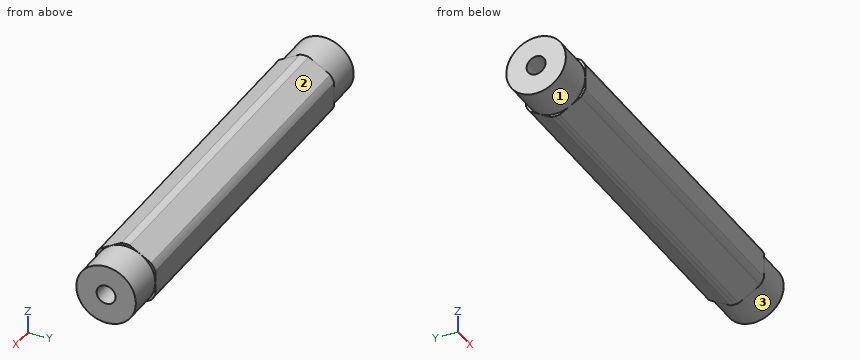
```python
from build123d import *

# Parameters (mm, degrees)
SKETCH1_R               = 2.0193
BOSS_EXTRUDE1_DEPTH     = 44.45
SKETCH2_R               = 8.89
SKETCH2_R_2             = 6.35
CUT_EXTRUDE_THIN1_DEPTH = 7.9375


with BuildPart() as part:
    # Sketch1 → Boss-Extrude1 (new, symmetric)
    with BuildSketch(Plane(origin=(0, 0, 0), x_dir=(0, 0, -1), z_dir=(1, 0, 0))):
        with BuildLine():
            ThreePointArc((6.874999966, 0), (6.860422465, 0.447468582), (6.816751782, 0.893039571))
            Line((6.816751782, 0.893039571), (4.181770846, 5.456960429))
            ThreePointArc((4.181770846, 5.456960429), (3.437499983, 5.953924622), (2.634980936, 6.35))
            Line((2.634980936, 6.35), (-2.634980936, 6.35))
            ThreePointArc((-2.634980936, 6.35), (-3.437499983, 5.953924622), (-4.181770846, 5.456960429))
            Line((-4.181770846, 5.456960429), (-6.816751782, 0.893039571))
            ThreePointArc((-6.816751782, 0.893039571), (-6.874999966, 0), (-6.816751782, -0.893039571))
            Line((-6.816751782, -0.893039571), (-4.181770846, -5.456960429))
            ThreePointArc((-4.181770846, -5.456960429), (-3.437499983, -5.953924622), (-2.634980936, -6.35))
            Line((-2.634980936, -6.35), (2.634980936, -6.35))
            ThreePointArc((2.634980936, -6.35), (3.437499983, -5.953924622), (4.181770846, -5.456960429))
            Line((4.181770846, -5.456960429), (6.816751782, -0.893039571))
            ThreePointArc((6.816751782, -0.893039571), (6.860422465, -0.447468582), (6.874999966, 0))
        make_face()
        Circle(SKETCH1_R, mode=Mode.SUBTRACT)
    extrude(amount=BOSS_EXTRUDE1_DEPTH, both=True)

    # Sketch2 → Cut-Extrude-Thin1 (cut)
    with BuildSketch(Plane(origin=(44.45, 0, 0), x_dir=(0, 0, -1), z_dir=(1, 0, 0))):
        Circle(SKETCH2_R)
        Circle(SKETCH2_R_2, mode=Mode.SUBTRACT)
    cut_extrude_thin1 = extrude(amount=-CUT_EXTRUDE_THIN1_DEPTH, mode=Mode.SUBTRACT)

    # Mirror1: Cut-Extrude-Thin1 across plane
    add(cut_extrude_thin1.mirror(Plane(origin=(0, 0, 0), x_dir=(0, 0, 1), z_dir=(1, 0, 0))), mode=Mode.SUBTRACT)


solid = part.part
```
Model file for the job. Use its own axes, mm. Face numbers are marked on the shaded views. A direction names the side the tool comes from. Give positions to 0.01 mm unless a question says otherwise; leave off trailing zeros. Write each loop counter-clockwise with the first axis right and the second up, starting at its lowest first coordinate (ties: lowest second). Pieces come first, ordered by that corner, then holes. Notation, with made-up numbers: M -8.75,36 L 28.25,36 A16 cw 28.25,57 Z; hole C -13,26 d5. An arc over 180 degrees is marked long. Use a Markdown table: item, result.
1) Pin check, flat tips, straight feed: pin 1 (1 mm diameter, centred on x = 18.5, z = 4.5, fed in from -Y); pin 2 (1 mm diameter, centred on x = -2.5, y = 1, fed in from +Z). Stop position of each tip, or through.
Responses:
| item | result |
|---|---|
| pin 1 | stops at y = -5.59 |
| pin 2 | stops at z = 6.86 |
2) Tool access for the marked faces 1, 2 and 3: list every direction of +Z, -Z, +X, -X, +Y, -Y with a clear straight run to the whole face (end or side of a thin tool).
Responses:
| item | result |
|---|---|
| face 1 | -X |
| face 2 | +Z, +X, -X, +Y |
| face 3 | +X |
3) Cut at B-B (y = 4.25). List the corners of the cut face in (x, z), and give its area (3 significant figures).
Responses:
| item | result |
|---|---|
| outline | M -44.45,-4.72 L -36.51,-4.72 L -36.51,-4.88 L 36.51,-4.88 L 36.51,-4.72 L 44.45,-4.72 L 44.45,4.72 L 36.51,4.72 L 36.51,4.88 L -36.51,4.88 L -36.51,4.72 L -44.45,4.72 Z |
| area | 862 mm2 |
4) Drill centre lines: line 1 (Z direction, x = 24.5, y = 0.25); line 2 (Z direction, x = 12, y = 1) (3 decimals); line 3 (Y direction, x = -31, z = -1.75). Where is each one in solid material? Low to high. Write a range as from..to.
Responses:
| item | result |
|---|---|
| line 1 | z = -6.87..-2, 2..6.87 |
| line 2 | z = -6.755..-1.754, 1.754..6.755 |
| line 3 | y = -6.35..-1.01, 1.01..6.35 |
5) Cut at A-A (x = -16). List the corners of the cut face in (y, z) (3 decimals).
Responses:
| item | result |
|---|---|
| outline | M -6.35,-2.635 A6.875 ccw -5.457,-4.182 L -0.893,-6.817 A6.875 ccw 0.893,-6.817 L 5.457,-4.182 A6.875 ccw 6.35,-2.635 L 6.35,2.635 A6.875 ccw 5.457,4.182 L 0.893,6.817 A6.875 ccw -0.893,6.817 L -5.457,4.182 A6.875 ccw -6.35,2.635 Z; hole C 0,0 d4.039 |
